Input: dimensioned drawing with shaded views. Units: mm. Origin: part minimum x, y, z. Coordinates: 2 decimals unless noted, no trailing zeros. Order: outer loops, then holes, each group sorted by start corner. A loop starts at its lowest first (then second) coordinate and runs counter-clockwise, first axis right, second up. Notation, with made-up numbers: M 0,23 L 14,23 A9 ccw 14,32 Z; hole C -30.5,5.25 d7. An arc over 180 degrees is marked long. Use CSV: the item, a comma, the result in double quotes. Start each with the question number.
1. Pull-direction query (Z, two-part tool) for the marked faces 1, 2, 3 and 4; classes: pulls with the +Z half, pulls with the -Z half, needs draft (parallel to the pull), parting line crosses it, or undercut.
2. Section query D-D on x = 8. Return the cut outline in (y, z).
3. Section query B-B on x = 25. Return the cut outline in (y, z), and give its area (3 significant figures).
4. Section query A-A on y = 0.85. Return the cut outline in (x, z), and give its area (3 significant figures).
5. Material intervals for line 1 (Z direction, x = 65, y = 2.05); line 2 (Y direction, x = 48, z = 8.5); line 3 (X direction, y = 2.75, z = 13), sorted ascending.
6. Section query C-C on z = 18. Return the cut outline in (x, y).
7. First-contact query: P1, Ø3, axis at y = 4.5, z = 4, coming from the -X side; P2, Ø2, axis at x = 4.5, y = 1, coming from the -Z side; P3, Ø2, axis at y = 4.5, z = 35, coming from the -X side. Flat tips, straight axial feed; report the tip coordinate or a pass-through.
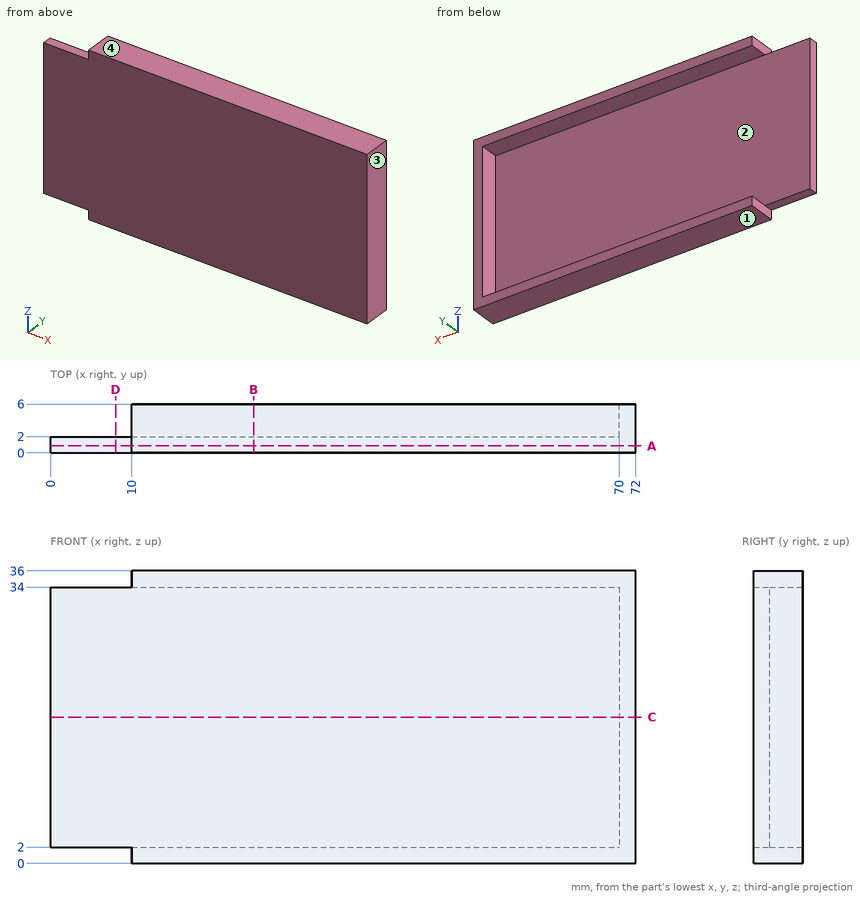
Results list:
1,face 1,"pulls with the -Z half"
1,face 2,"undercut"
1,face 3,"needs draft"
1,face 4,"pulls with the +Z half"
2,outline,"M 0,2 L 2,2 L 2,34 L 0,34 Z"
3,outline,"M 0,0 L 6,0 L 6,2 L 2,2 L 2,34 L 6,34 L 6,36 L 0,36 Z"
3,area,"88.0 mm²"
4,outline,"M 0,2 L 10,2 L 10,0 L 72,0 L 72,36 L 10,36 L 10,34 L 0,34 Z"
4,area,"2,550 mm²"
5,line 1,"z = 0 to 2, 34 to 36"
5,line 2,"y = 0 to 2"
5,line 3,"x = 70 to 72"
6,outline,"M 0,0 L 72,0 L 72,6 L 70,6 L 70,2 L 0,2 Z"
7,P1,"stops at x = 70"
7,P2,"stops at z = 2"
7,P3,"stops at x = 10"
